from build123d import *

# Parameters (mm, degrees)
SKETCH3_R          = 1
CUT_EXTRUDE1_DEPTH = 3
CUT_EXTRUDE2_START = -4
SKETCH4_R          = 1
CUT_EXTRUDE2_DEPTH = 4
CUT_EXTRUDE3_START = -3
CUT_EXTRUDE3_DEPTH = 3
CUT_EXTRUDE4_DEPTH = 3


with BuildPart() as part:
    # Sketch1 → Revolve1 (revolve)
    with BuildSketch(Plane(origin=(0, 0, 0), x_dir=(0, 0, -1), z_dir=(1, 0, 0)), mode=Mode.PRIVATE) as revolve1_sk:
        Polygon((0, 18.5), (-0.75, 18.5), (-0.75, 14.5), (-6.392893219, 14.5), (-7.1, 13.792893219), (-7.1, 0), (-1, 0), (-1, -1), (0, -1), (0, 0), align=None)
    revolve(revolve1_sk.sketch.rotate(Axis((0, 0, 0), (0, 1, 0)), 180), axis=Axis((0, 0, 0), (0, 1, 0)))

    # Sketch3 → Cut-Extrude1 (cut)
    with BuildSketch(Plane.XZ):
        with Locations(Location((0, 4.5, 0), (0, 0, 270))):
            Circle(SKETCH3_R)
        with Locations(Location((4.5, 0, 0), (0, 0, 270))):
            Circle(SKETCH3_R)
        with Locations(Location((-4.5, 0, 0), (0, 0, 270))):
            Circle(SKETCH3_R)
        with Locations(Location((0, -4.5, 0), (0, 0, 270))):
            Circle(SKETCH3_R)
    extrude(amount=-CUT_EXTRUDE1_DEPTH, mode=Mode.SUBTRACT)

    # Sketch4 → Cut-Extrude2 (cut)
    with BuildSketch(Plane(origin=(0, 14.5, 0), x_dir=(1, 0, 0), z_dir=(0, 1, 0)).offset(CUT_EXTRUDE2_START)):
        with Locations(Location((0, 4.5, 0), (0, 0, 90))):
            Circle(SKETCH4_R)
        with Locations(Location((2.5, 0, 0), (0, 0, 270))):
            Circle(SKETCH4_R)
        with Locations(Location((0, -4.5, 0), (0, 0, 90))):
            Circle(SKETCH4_R)
        with Locations(Location((-2.5, 0, 0), (0, 0, 270))):
            Circle(SKETCH4_R)
    extrude(amount=CUT_EXTRUDE2_DEPTH, mode=Mode.SUBTRACT)

    # Sketch5 → Cut-Extrude3 (cut)
    with BuildSketch(Plane(origin=(0, 14.5, 0), x_dir=(1, 0, 0), z_dir=(0, 1, 0)).offset(CUT_EXTRUDE3_START)):
        with BuildLine():
            ThreePointArc((-2.7, 6.566582064), (0, 7.1), (2.7, 6.566582064))
            add(Edge.make_bspline(
                [(-2.7, 6.566582064), (-2.071231518, 5.5), (0, 6.5), (2.071231518, 5.5), (2.7, 6.566582064)],
                knots=[0, 0, 0, 0, 0, 1, 1, 1, 1, 1], degree=4))
        make_face()
        with BuildLine():
            ThreePointArc((4.336826883, 5.621559622), (6.148780367, 3.55), (7.036826883, 0.945022442))
            add(Edge.make_bspline(
                [(4.336826883, 5.621559622), (3.727523962, 4.543739111), (5.629165125, 3.25), (5.79875548, 0.956260889), (7.036826883, 0.945022442)],
                knots=[0, 0, 0, 0, 0, 1, 1, 1, 1, 1], degree=4))
        make_face()
        with BuildLine():
            ThreePointArc((7.036826883, -0.945022442), (6.148780367, -3.55), (4.336826883, -5.621559622))
            add(Edge.make_bspline(
                [(7.036826883, -0.945022442), (5.79875548, -0.956260889), (5.629165125, -3.25), (3.727523962, -4.543739111), (4.336826883, -5.621559622)],
                knots=[0, 0, 0, 0, 0, 1, 1, 1, 1, 1], degree=4))
        make_face()
        with BuildLine():
            ThreePointArc((2.7, -6.566582064), (0, -7.1), (-2.7, -6.566582064))
            add(Edge.make_bspline(
                [(2.7, -6.566582064), (2.071231518, -5.5), (0, -6.5), (-2.071231518, -5.5), (-2.7, -6.566582064)],
                knots=[0, 0, 0, 0, 0, 1, 1, 1, 1, 1], degree=4))
        make_face()
        with BuildLine():
            ThreePointArc((-4.336826883, -5.621559622), (-6.148780367, -3.55), (-7.036826883, -0.945022442))
            add(Edge.make_bspline(
                [(-4.336826883, -5.621559622), (-3.727523962, -4.543739111), (-5.629165125, -3.25), (-5.79875548, -0.956260889), (-7.036826883, -0.945022442)],
                knots=[0, 0, 0, 0, 0, 1, 1, 1, 1, 1], degree=4))
        make_face()
        with BuildLine():
            ThreePointArc((-7.036826883, 0.945022442), (-6.148780367, 3.55), (-4.336826883, 5.621559622))
            add(Edge.make_bspline(
                [(-7.036826883, 0.945022442), (-5.79875548, 0.956260889), (-5.629165125, 3.25), (-3.727523962, 4.543739111), (-4.336826883, 5.621559622)],
                knots=[0, 0, 0, 0, 0, 1, 1, 1, 1, 1], degree=4))
        make_face()
    extrude(amount=CUT_EXTRUDE3_DEPTH, mode=Mode.SUBTRACT)

    # Sketch6 → Cut-Extrude4 (cut)
    with BuildSketch(Plane.XZ):
        with BuildLine():
            Line((-1.718410499, 6.888908866), (-1.718410499, 3.486177452))
            Line((-1.718410499, 3.486177452), (-3.486177452, 1.718410499))
            Line((-3.486177452, 1.718410499), (-6.888908866, 1.718410499))
            ThreePointArc((-6.888908866, 1.718410499), (-5.020458146, 5.020458146), (-1.718410499, 6.888908866))
        make_face()
        with BuildLine():
            Line((1.718410499, 3.486177452), (1.718410499, 6.888908866))
            ThreePointArc((1.718410499, 6.888908866), (5.020458146, 5.020458146), (6.888908866, 1.718410499))
            Line((6.888908866, 1.718410499), (3.486177452, 1.718410499))
            Line((3.486177452, 1.718410499), (1.718410499, 3.486177452))
        make_face()
        with BuildLine():
            Line((3.486177452, -1.718410499), (6.888908866, -1.718410499))
            ThreePointArc((6.888908866, -1.718410499), (5.020458146, -5.020458146), (1.718410499, -6.888908866))
            Line((1.718410499, -6.888908866), (1.718410499, -3.486177452))
            Line((1.718410499, -3.486177452), (3.486177452, -1.718410499))
        make_face()
        with BuildLine():
            Line((-1.718410499, -3.486177452), (-1.718410499, -6.888908866))
            ThreePointArc((-1.718410499, -6.888908866), (-5.020458146, -5.020458146), (-6.888908866, -1.718410499))
            Line((-6.888908866, -1.718410499), (-3.486177452, -1.718410499))
            Line((-3.486177452, -1.718410499), (-1.718410499, -3.486177452))
        make_face()
    extrude(amount=-CUT_EXTRUDE4_DEPTH, mode=Mode.SUBTRACT)

    # Sketch7 → Cut-Revolve1 (revolve, cut)
    with BuildSketch(Plane(origin=(0, 0, 0), x_dir=(0, 0, -1), z_dir=(1, 0, 0)), mode=Mode.PRIVATE) as cut_revolve1_sk:
        Polygon((-7.1, 3.55), (-6.6, 3.8), (-6.6, 4.2), (-7.1, 4.45), align=None)
    revolve(cut_revolve1_sk.sketch.rotate(Axis((0, 0, 0), (0, 1, 0)), 180), axis=Axis((0, 0, 0), (0, 1, 0)), mode=Mode.SUBTRACT)


solid = part.part
Read the model definition and answer for the solid it produces. Units are mm, in the model's axes. A direction names the side the tool comes from. Coordinates: 2 decimals unless noted, no trailing zeros. Loops run counter-clockwise (first coordinate to the right, second up) from the corner with the lowest first, then second, coordinate; pieces in that order, holes last. Notation, with made-up numbers: (-7, 67) - (17, 67) arc R24 ccw to (17, 98) - close; hole circle Ø7 at (67, 72.5). An arc over 180 degrees is marked (long way). Answer in a Markdown table with one row per item.
Q1. For faces 5 (the flat face through (-2, 10.5, 0)), 6 (the cylindrical face through (-0.6, 1.5, 5.3)), 7 (the flat face through (4, 3, -4)), determine the directions among +Z, -Z, +X, -X, +Y, -Y from which every point of the face is accessible in a straight line to the end or side of a thin tool.
Here are the results:
| item | result |
|---|---|
| face 5 | +Y |
| face 6 | -Y |
| face 7 | -Z, +X, -Y |
Q2. Given P1, Ø1.4, axis at x = -6, z = 3.5, coming from the +Y side; P2, Ø5, axis at x = 4.5, y = 9, coming from the -Z side; P3, Ø2.5, axis at x = 0, z = -4.5, coming from the -Y side; P4, Ø5, axis at x = 1, y = 5.5, coming from the +Z side, each flat-ended and moving along its own axis, determine where each tip first touches the part or whether it passes through.
Here are the results:
| item | result |
|---|---|
| P1 | stops at y = 11.5 |
| P2 | stops at z = -6.81 |
| P3 | stops at y = 0 |
| P4 | stops at z = 7.1 |
Q3. Straight lines are drawn through the part: line 1 along X through (y, z) = (12.25, 0); line 2 along X through (y, z) = (0.8, 0); line 3 along X through (y, z) = (1.25, 4.5). For each, find the intervals that lie inside material, in ascending order. Write a range as [from, to].
Here are the results:
| item | result |
|---|---|
| line 1 | x = [-7.1, -3.5], [-1.5, 1.5], [3.5, 7.1] |
| line 2 | x = [-7.1, -5.5], [-3.5, 3.5], [5.5, 7.1] |
| line 3 | x = [-1.72, -1], [1, 1.72] |
Q4. The mould has two halves that part along Y. Classify faces 1 (the flat face through (-6, 11.5, -3)), 2 (the cylindrical face through (-4.461, 4.003, 4.864)), 3 (the flat face through (0, 3, 5)), 4 (the flat face through (-1.718, 1, 5)): pulls with the +Y half, pulls with the -Y half, needs draft (parallel to the pull), parting line crosses it, or undercut.
Here are the results:
| item | result |
|---|---|
| face 1 | pulls with the +Y half |
| face 2 | undercut |
| face 3 | pulls with the -Y half |
| face 4 | needs draft |
Q5. Find section A-A on y = 1. Write down the section's boundary in (x, z).
Here are the results:
| item | result |
|---|---|
| outline | (-6.89, -1.72) - (-3.49, -1.72) - (-1.72, -3.49) - (-1.72, -6.89) arc R7.1 ccw to (1.72, -6.89) - (1.72, -3.49) - (3.49, -1.72) - (6.89, -1.72) arc R7.1 ccw to (6.89, 1.72) - (3.49, 1.72) - (1.72, 3.49) - (1.72, 6.89) arc R7.1 ccw to (-1.72, 6.89) - (-1.72, 3.49) - (-3.49, 1.72) - (-6.89, 1.72) arc R7.1 ccw to start; hole circle Ø2 at (-4.5, 0); hole circle Ø2 at (0, -4.5); hole circle Ø2 at (0, 4.5); hole circle Ø2 at (4.5, 0) |
Q6. Find section B-B on y = 15.75. Write down the section's boundary in (x, z).
Here are the results:
| item | result |
|---|---|
| outline | circle Ø1.5 at (0, 0) |
Q7. Find section C-C on y = 11.75. Count the separate pieces of the cut face and the enclosed holes in it, plus the area to 3 significant figures.
Here are the results:
| item | result |
|---|---|
| separate pieces | 1 |
| enclosed holes | 4 |
| area | 119 mm^2 |
